from build123d import *

# Parameters (mm, degrees)
SKETCH1_R               = 6.35
BOSS_EXTRUDE1_DEPTH     = 5.4
HORN_DEPTH              = 2.5
SKETCH4_R               = 1.4
CUT_EXTRUDE1_DEPTH      = 6.4
SKETCH5_R               = 0.5
CUT_EXTRUDE2_DEPTH      = 6.4
LPATTERN1_COUNT         = 4
LPATTERN1_PITCH         = 3
MIRROR1_COPY_1_SKETCH_R = 0.5
MIRROR1_COPY_1_DEPTH    = 6.4
MIRROR1_COPY_2_SKETCH_R = 0.5
MIRROR1_COPY_2_DEPTH    = 6.4
MIRROR1_COPY_3_SKETCH_R = 0.5
MIRROR1_COPY_3_DEPTH    = 6.4
CUT_EXTRUDE4_DEPTH      = 3
CIRPATTERN2_COUNT       = 26
SKETCH9_R               = 2.6
CUT_EXTRUDE5_DEPTH      = 3
SKETCH10_R              = 6.35
SKETCH10_R_2            = 4.25
CUT_EXTRUDE6_DEPTH      = 2.9
BOSS_EXTRUDE5_DEPTH     = 0.5
CIRPATTERN3_COUNT       = 4
SKETCH12_R              = 4.375
CUT_EXTRUDE7_DEPTH      = 1
SKETCH13_R              = 3.375
SKETCH13_R_2            = 2.875
BOSS_EXTRUDE6_DEPTH     = 1
SKETCH14_R              = 3.375
SKETCH14_R_2            = 2.875
BOSS_EXTRUDE7_DEPTH     = 0.35
CUT_EXTRUDE8_DEPTH      = 6.4


with BuildPart() as part:
    # Sketch1 → Boss-Extrude1 (new body)
    with BuildSketch(Plane(origin=(0, 0, 0), x_dir=(1, 0, 0), z_dir=(0, 1, 0))):
        Circle(SKETCH1_R)
    extrude(amount=BOSS_EXTRUDE1_DEPTH)

    # Sketch2 → horn (add)
    with BuildSketch(Plane(origin=(0, 5.4, 0), x_dir=(1, 0, 0), z_dir=(0, 1, 0))):
        with BuildLine():
            Line((-2.609740545, 16.990167671), (-4.891612682, 4.049027706))
            ThreePointArc((-4.891612682, 4.049027706), (0, 6.35), (4.891612682, 4.049027706))
            Line((4.891612682, 4.049027706), (2.609740545, 16.990167671))
            ThreePointArc((2.609740545, 16.990167671), (0, 19.18), (-2.609740545, 16.990167671))
        make_face()
    horn = extrude(amount=-HORN_DEPTH)

    # Sketch4 → Cut-Extrude1 (cut, through all)
    with BuildSketch(Plane(origin=(0, 5.4, 0), x_dir=(-1, 0, 0), z_dir=(0, -1, 0))):
        Circle(SKETCH4_R)
    extrude(amount=CUT_EXTRUDE1_DEPTH, mode=Mode.SUBTRACT)

    # Sketch5 → Cut-Extrude2 (cut, through all)
    with BuildSketch(Plane(origin=(0, 0, 0), x_dir=(-1, 0, 0), z_dir=(0, -1, 0))):
        with Locations((0, 16.53)):
            Circle(SKETCH5_R)
    cut_extrude2 = extrude(amount=-CUT_EXTRUDE2_DEPTH, mode=Mode.SUBTRACT)

    # LPattern1: Cut-Extrude2 ×4
    with Locations(*[(0, 0, i * LPATTERN1_PITCH) for i in range(1, LPATTERN1_COUNT)]):
        add(cut_extrude2, mode=Mode.SUBTRACT)

    # Mirror1: horn, Cut-Extrude2 across plane
    add(horn.mirror(Plane.XY))
    add(cut_extrude2.mirror(Plane.XY), mode=Mode.SUBTRACT)

    # Mirror1 copy 1 sketch → Mirror1 copy 1 (cut, through all)
    with BuildSketch(Plane(origin=(0, 0, -3), x_dir=(-1, 0, 0), z_dir=(0, -1, 0))):
        with Locations((0, -16.53)):
            Circle(MIRROR1_COPY_1_SKETCH_R)
    extrude(amount=-MIRROR1_COPY_1_DEPTH, mode=Mode.SUBTRACT)

    # Mirror1 copy 2 sketch → Mirror1 copy 2 (cut, through all)
    with BuildSketch(Plane(origin=(0, 0, -6), x_dir=(-1, 0, 0), z_dir=(0, -1, 0))):
        with Locations((0, -16.53)):
            Circle(MIRROR1_COPY_2_SKETCH_R)
    extrude(amount=-MIRROR1_COPY_2_DEPTH, mode=Mode.SUBTRACT)

    # Mirror1 copy 3 sketch → Mirror1 copy 3 (cut, through all)
    with BuildSketch(Plane(origin=(0, 0, -9), x_dir=(-1, 0, 0), z_dir=(0, -1, 0))):
        with Locations((0, -16.53)):
            Circle(MIRROR1_COPY_3_SKETCH_R)
    extrude(amount=-MIRROR1_COPY_3_DEPTH, mode=Mode.SUBTRACT)

    # Sketch8 → Cut-Extrude4 (cut)
    with BuildSketch(Plane(origin=(0, 0, 0), x_dir=(-1, 0, 0), z_dir=(0, -1, 0))):
        with BuildLine():
            Line((0, -2.9), (0.262912611, -2.586672952))
            ThreePointArc((0.262912611, -2.586672952), (0, -2.6), (-0.262912611, -2.586672952))
            Line((-0.262912611, -2.586672952), (0, -2.9))
        make_face()
    cut_extrude4 = extrude(amount=-CUT_EXTRUDE4_DEPTH, mode=Mode.SUBTRACT)

    # CirPattern2: Cut-Extrude4 ×26 about axis
    cirpattern2_axis = Axis((0, 0, 0), (0, 1, 0))
    for i in range(1, CIRPATTERN2_COUNT):
        add(cut_extrude4.rotate(cirpattern2_axis, i * 360 / CIRPATTERN2_COUNT), mode=Mode.SUBTRACT)

    # Sketch9 → Cut-Extrude5 (cut)
    with BuildSketch(Plane(origin=(0, 0, 0), x_dir=(-1, 0, 0), z_dir=(0, -1, 0))):
        Circle(SKETCH9_R)
    extrude(amount=-CUT_EXTRUDE5_DEPTH, mode=Mode.SUBTRACT)

    # Sketch10 → Cut-Extrude6 (cut)
    with BuildSketch(Plane(origin=(0, 0, 0), x_dir=(-1, 0, 0), z_dir=(0, -1, 0))):
        Circle(SKETCH10_R)
        Circle(SKETCH10_R_2, mode=Mode.SUBTRACT)
    extrude(amount=-CUT_EXTRUDE6_DEPTH, mode=Mode.SUBTRACT)

    # Sketch11 → Boss-Extrude5 (add, symmetric)
    with BuildSketch(Plane.XY):
        Polygon((4.21, 0.99), (5.812680296, 2.9), (4.21, 2.9), (4.16, 2.9), (4.16, 0.99), align=None)
    boss_extrude5 = extrude(amount=BOSS_EXTRUDE5_DEPTH, both=True)

    # CirPattern3: Boss-Extrude5 ×4 about axis
    cirpattern3_axis = Axis((0, 0, 0), (0, 1, 0))
    for i in range(1, CIRPATTERN3_COUNT):
        add(boss_extrude5.rotate(cirpattern3_axis, i * 360 / CIRPATTERN3_COUNT))

    # Sketch12 → Cut-Extrude7 (cut)
    with BuildSketch(Plane(origin=(0, 5.4, 0), x_dir=(1, 0, 0), z_dir=(0, 1, 0))):
        Circle(SKETCH12_R)
    extrude(amount=-CUT_EXTRUDE7_DEPTH, mode=Mode.SUBTRACT)

    # Sketch13 → Boss-Extrude6 (add)
    with BuildSketch(Plane(origin=(0, 4.4, 0), x_dir=(1, 0, 0), z_dir=(0, 1, 0))):
        Circle(SKETCH13_R)
        Circle(SKETCH13_R_2, mode=Mode.SUBTRACT)
    extrude(amount=BOSS_EXTRUDE6_DEPTH)

    # Sketch14 → Boss-Extrude7 (add)
    with BuildSketch(Plane(origin=(0, 5.4, 0), x_dir=(1, 0, 0), z_dir=(0, 1, 0))):
        Circle(SKETCH14_R)
        Circle(SKETCH14_R_2, mode=Mode.SUBTRACT)
    extrude(amount=BOSS_EXTRUDE7_DEPTH)

    # Sketch15 → Cut-Extrude8 (cut, through all)
    with BuildSketch(Plane(origin=(0, 5.4, 0), x_dir=(1, 0, 0), z_dir=(0, 1, 0))):
        Polygon((-3.616359732, -11.281346581), (3.616359732, -11.281346581), (9.32149419, -16.388605274), (4.660747095, -20.846711191), (-5.775273574, -20.846711191), (-10.680070262, -15.7189692), (-9.733647563, -14.813695314), align=None)
    extrude(amount=-CUT_EXTRUDE8_DEPTH, mode=Mode.SUBTRACT)


solid = part.part
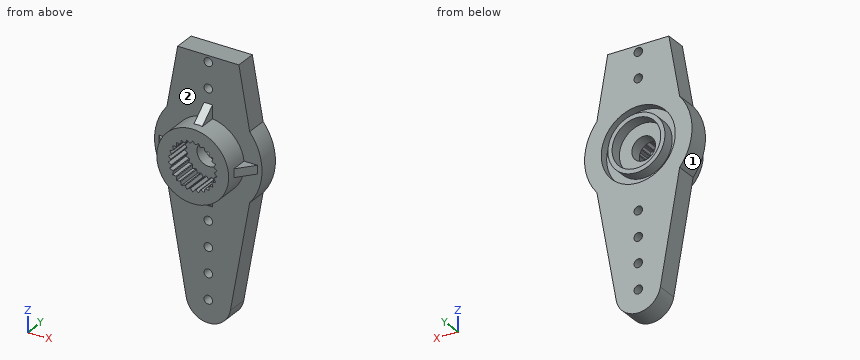
Here's how the part is built. I have some questions about the finished solid (model axes, mm). Face numbers are marked on the shaded views. A direction names the side the tool comes from. Round coordinates to 2 decimals unless told otherwise and drop trailing zeros. Order: outer loops, then holes, each group sorted by start corner. A loop starts at its lowest first (then second) coordinate and runs counter-clockwise, first axis right, second up. Notation, with made-up numbers: (82, 19) -> (113, 19) arc R19 cw to (113, 41) -> close; hole circle Ø1 at (74, 66.5). An arc over 180 degrees is marked (long way). Return JSON: item names as keys, results as strings.
Q1. If we section it at A-A on y = 4.8: Give the number of separate pieces and of enclosed holes in the cut face, plus the area to 3 significant figures.
Filled sheet:
{"separate pieces": "2", "enclosed holes": "8", "area": "208 mm^2"}
Q2. Which directions (+Z, -Z, +X, -X, +Y, -Y) give clear straight access to the entire face, cutting with the end or side of a thin tool? Please do the marked faces 1 and 2.
Filled sheet:
{"face 1": "-X, +Y, -Y", "face 2": "-Y"}
Q3. For pin 1 Ø0.5 at (y, z) = (2, -5) entering from -X; pin 2 Ø0.8 at (x, y) = (-5, 1.5) entering from +Z; pin 3 Ø1.7 at (x, z) = (0, 0) entering from -Y; pin 4 Ø1.5 at (y, z) = (4.5, 3.5) entering from -X, each with a flat end and sliding along its axis, tell me the tip position at first contact or that it passes through.
Filled sheet:
{"pin 1": "stops at x = -0.5", "pin 2": "stops at z = 0.5", "pin 3": "passes through", "pin 4": "stops at x = -5.72"}
Q4. If we section it at C-C on x = 5.25: List the corners of the cut face in (y, z) for me.
Filled sheet:
{"outline": "(2.23, -0.5) -> (2.9, -0.5) -> (2.9, -3.57) -> (5.4, -3.57) -> (5.4, 3.57) -> (2.9, 3.57) -> (2.9, 0.5) -> (2.23, 0.5) -> close"}
Q5. If we section it at D-D on z = -13.53: List the corners of the cut face in (x, y) for me, plus the area to 3 significant figures.
Filled sheet:
{"outline": "(-3.22, 2.9) -> (-0.5, 2.9) -> (-0.5, 5.4) -> (-3.22, 5.4) -> close; (0.5, 2.9) -> (3.22, 2.9) -> (3.22, 5.4) -> (0.5, 5.4) -> close", "area": "13.6 mm^2"}
Q6. If we section it at B-B on z = 10.53: List the corners of the cut face in (x, y) for me, plus the area to 3 significant figures.
Filled sheet:
{"outline": "(-3.75, 2.9) -> (-0.5, 2.9) -> (-0.5, 5.4) -> (-3.75, 5.4) -> close; (0.5, 2.9) -> (3.75, 2.9) -> (3.75, 5.4) -> (0.5, 5.4) -> close", "area": "16.2 mm^2"}
Q7. I need wall thicknesses on line 1 along X through (y, z) = (5.15, 0) (3 decimals); line 2 along X through (y, z) = (2.65, -2.5); line 3 along Y through (x, z) = (3.5, 3). Which ranges of each line are inside material? Lowest first, please. Write a range as from..to.
Filled sheet:
{"line 1": "x = -6.35..-4.375, -3.375..-2.875, 2.875..3.375, 4.375..6.35", "line 2": "x = -3.44..-1.36, -1.18..-0.85, 0.85..1.18, 1.36..3.44", "line 3": "y = 2.9..5.4"}
